Model file for the job. Use its own axes, mm. Face numbers are marked on the shaded views. A direction names the side the tool comes from. Round coordinates to 2 decimals unless told otherwise and drop trailing zeros. Loops run counter-clockwise (first coordinate to the right, second up) from the corner with the lowest first, then second, coordinate; pieces in that order, holes last. Notation, with made-up numbers: (-12, 84) -> (42, 84) arc R23 ccw to (42, 101) -> close; hole circle Ø3 at (54, -10.75). An arc over 180 degrees is marked (long way). Use a Markdown table: item, result.
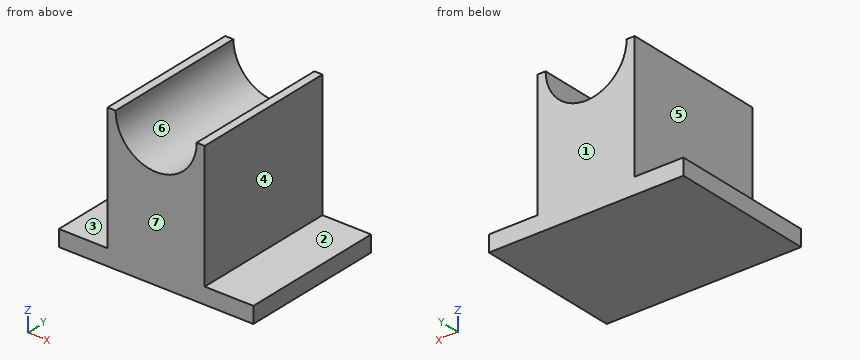
from build123d import *

# Parameters (mm, degrees)
F1_DEPTH = 114.3
F3_DEPTH = 114.301


with BuildPart() as f1:
    # F0 (on Front) → F1 (new body)
    with BuildSketch(Plane.XZ):
        Polygon((0, 12.7), (0, 0), (152.4, 0), (152.4, 12.7), (114.3, 12.7), (114.3, 111.125), (38.1, 111.125), (38.1, 12.7), align=None)
    extrude(amount=F1_DEPTH)

    # F2 (on face) → F3 (cut, through all)
    with BuildSketch(Plane.XZ.offset(114.3)):
        with BuildLine():
            Line((107.95, 111.125), (44.45, 111.125))
            ThreePointArc((44.45, 111.125), (76.2, 79.375), (107.95, 111.125))
        make_face()
    extrude(amount=-F3_DEPTH, mode=Mode.SUBTRACT)


solid = f1.part
Q1. Flat gauge pins, fed straight in: pin 1 (11.5 mm diameter, centred on x = 131, y = -55.5, fed in from +Z); pin 2 (3 mm diameter, centred on x = 61, y = -95.5, fed in from -Z); pin 3 (3 mm diameter, centred on x = 56, y = -64, fed in from +Z); pin 4 (12 mm diameter, centred on y = -67, z = 27, fed in from -X). Where does each tip first touch, or does it go through?
Results list:
| item | result |
|---|---|
| pin 1 | stops at z = 12.7 |
| pin 2 | stops at z = 0 |
| pin 3 | stops at z = 87.95 |
| pin 4 | stops at x = 38.1 |
Q2. Band-saw the part on B-B, the plane z = 95. Give the cut face in (x, y), plus the area to 3 significant figures.
Results list:
| item | result |
|---|---|
| outline | (38.1, -114.3) -> (48.85, -114.3) -> (48.85, 0) -> (38.1, 0) -> close; (103.55, -114.3) -> (114.3, -114.3) -> (114.3, 0) -> (103.55, 0) -> close |
| area | 2,460 mm² |
Q3. Pull direction X, two halves, no side cores. Call the marked faces 4, 5, 6 and 7: released by +X, released by -X, zero draft, split by the parting line, or undercut.
Results list:
| item | result |
|---|---|
| face 4 | released by +X |
| face 5 | released by -X |
| face 6 | undercut |
| face 7 | zero draft |
Q4. Band-saw the part on A-A, the plane y = -79.5. Give the cut face in (x, z) (3 decimals), plus the area to 3 significant figures.
Results list:
| item | result |
|---|---|
| outline | (0, 0) -> (152.4, 0) -> (152.4, 12.7) -> (114.3, 12.7) -> (114.3, 111.125) -> (107.95, 111.125) arc R31.75 cw to (44.45, 111.125) -> (38.1, 111.125) -> (38.1, 12.7) -> (0, 12.7) -> close |
| area | 7,850 mm² |
Q5. Tool access for the marked faces 1, 2 and 3: list every direction of +Z, -Z, +X, -X, +Y, -Y with a clear straight run to the whole face (end or side of a thin tool).
Results list:
| item | result |
|---|---|
| face 1 | +Z, -Z, +X, -X, +Y |
| face 2 | +Z, +X, +Y, -Y |
| face 3 | +Z, -X, +Y, -Y |
Q6. Band-saw the part on D-D, the plane x = 123.5. Give the cut face in (y, z).
Results list:
| item | result |
|---|---|
| outline | (-114.3, 0) -> (0, 0) -> (0, 12.7) -> (-114.3, 12.7) -> close |
Q7. Drill centre lines: L1, parallel to Z at x = 129.5, y = -4.5; L2, parallel to X at y = -43.5, z = 27.5; L3, parallel to X at y = -77, z = 82. Where is each one in solid material? Low to high. Write a range as from..to.
Results list:
| item | result |
|---|---|
| L1 | z = 0..12.7 |
| L2 | x = 38.1..114.3 |
| L3 | x = 38.1..63.56, 88.84..114.3 |
Q8. Band-saw the part on C-C, the plane x = 76.2. Give the cut face in (y, z) (3 decimals), plus the area to 3 significant figures.
Results list:
| item | result |
|---|---|
| outline | (-114.3, 0) -> (0, 0) -> (0, 79.375) -> (-114.3, 79.375) -> close |
| area | 9,070 mm² |
